Geometry: final body of the model. Coordinates: model frame, mm. Face numbers are marked on the shaded views. Give positions to 0.01 mm unless a question says otherwise; leave off trailing zeros. Loops run counter-clockwise (first coordinate to the right, second up) from the corner with the lowest first, then second, coordinate; pieces in that order, holes last. Notation, with made-up numbers: M -19.75,17 L 13.25,17 A14 cw 13.25,31 Z; hole C 62,48 d3. An arc over 180 degrees is marked long. Put each result on its own line as item: value.
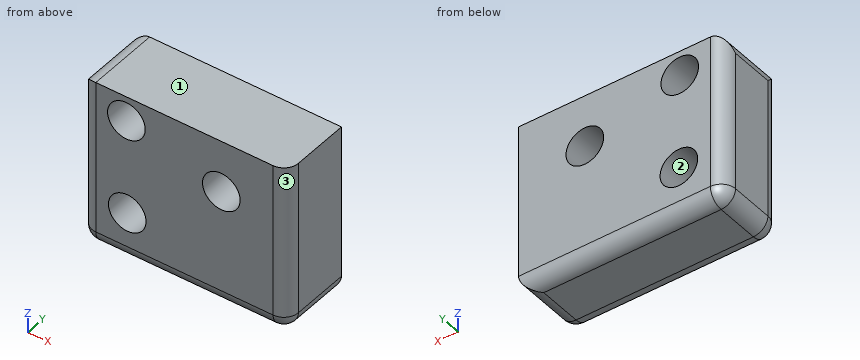
```python
from build123d import *

# Parameters (mm, degrees)
F0_W     = 71.305797
F0_H     = 58.31974
F1_DEPTH = 25
F3_D     = 13
F3_DEPTH = 51
F4_R     = 5


with BuildPart() as f1:
    # F0 (on Front) → F1 (new body)
    with BuildSketch(Plane.XZ):
        with Locations((-100.383364, 7.697545)):
            Rectangle(F0_W, F0_H)
    extrude(amount=F1_DEPTH)

    # F3
    with Locations(Plane.XZ.offset(25)):
        with Locations((-120.461434, 28.316814), (-120.157562, -4.412703), (-87.64419, 18.950811)):
            Hole(F3_D / 2, depth=F3_DEPTH)

    # F4
    f4_edges = [f1.edges().sort_by_distance(p)[0] for p in [
        (-64.730465, -25, 7.697545),
        (-100.383364, -25, -21.462325),
        (-136.036262, -12.5, -21.462325),
        (-64.730465, -12.5, -21.462325),
        (-100.383364, 0, -21.462325),
        (-136.036262, -12.5, 36.857415),
        (-136.036262, 0, 7.697545),
        (-136.036262, -25, 7.697545),
    ]]
    fillet(f4_edges, radius=F4_R)


solid = f1.part
```
Item 1: Line query: probe 1 along Z at (x, y) = (-116, -16.25); probe 2 along X at (y, z) = (-8.75, -1); probe 3 along X at (y, z) = (-17, 19). Output: solid intervals per line, ascending. Write a range as [from, to].
Output values:
probe 1: [-21.46, -9.41], [0.58, 23.59], [33.04, 36.86]
probe 2: [-136.04, -125.69], [-114.63, -64.73]
probe 3: [-136.04, -94.14], [-81.14, -64.73]
Item 2: Pin query (flat end, axial travel): pin 1 Ø15 at (x, z) = (-120.46, 28.32) entering from -Y; pin 2 Ø1.5 at (y, z) = (-21, 22) entering from -X. Return the tip coordinate at first contact, or that it passes through.
Output values:
pin 1: y = -25
pin 2: x = -136.03
Item 3: Section B-B on x = -122. Output: boundary loops of the cut face in (y, z).
Output values:
outline: M -25,-16.46 A5 ccw -20,-21.46 L -5,-21.46 A5 ccw 0,-16.46 L 0,-10.65 L -25,-10.65 Z; M -25,1.82 L 0,1.82 L 0,22 L -25,22 Z; M -25,34.63 L 0,34.63 L 0,36.86 L -25,36.86 Z
Item 4: Mould query, pull axis Z, two halves, no side actions, for the marked faces 1, 2 and 3. Classes: pulls with the +Z half, pulls with the -Z half, needs draft (parallel to the pull), parting line crosses it, or undercut.
Output values:
face 1: pulls with the +Z half
face 2: undercut
face 3: needs draft
Item 5: Section C-C on y = -22.75. Output: boundary loops of the cut face in (x, z), then the cut area to 3 significant figures.
Output values:
outline: M -135.21,-16.46 A4.18 ccw -131.04,-20.64 L -69.73,-20.64 A4.18 ccw -65.55,-16.46 L -65.55,36.86 L -131.04,36.86 A5 ccw -135.21,34.61 Z; hole C -120.46,28.32 d13; hole C -120.16,-4.41 d13; hole C -87.64,18.95 d13
area: 3,600 mm²
Item 6: Section D-D on z = 33. Output: boundary loops of the cut face in (x, y), then the cut area to 3 significant figures.
Output values:
outline: M -135.9,-21.14 A5 ccw -131.04,-25 L -124.97,-25 L -124.97,0 L -131.04,0 A5 ccw -135.9,-3.86 Z; M -115.95,-25 L -69.73,-25 A5 ccw -64.73,-20 L -64.73,0 L -115.95,0 Z
area: 1,540 mm²
Item 7: Section A-A on z = -6. Output: boundary loops of the cut face in (x, y).
Output values:
outline: M -136.04,-20 A5 ccw -131.04,-25 L -126.46,-25 L -126.46,0 L -131.04,0 A5 ccw -136.04,-5 Z; M -113.85,-25 L -69.73,-25 A5 ccw -64.73,-20 L -64.73,0 L -113.85,0 Z
